Check sheet for the drawn part. Datum: minimum x, y, z corner. Units: mm. A direction names the side the tool comes from. Give positions to 0.01 mm unless a question says otherwise; leave off trailing zeros. Write each loop counter-clockwise with the first axis right and the second up, starting at its lowest first coordinate (ties: lowest second). Pieces come first, ordered by that corner, then holes.
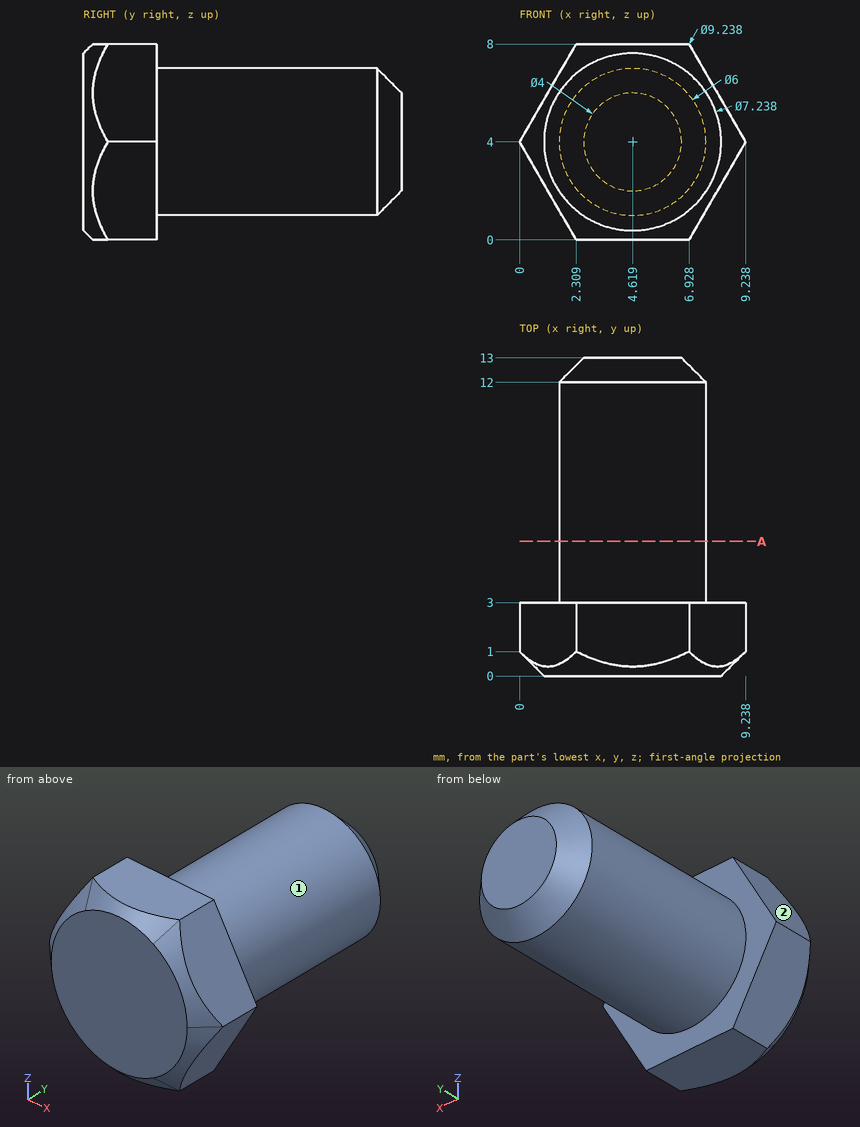
1) Access from +Z, -Z, +X, -X, +Y, -Y to the whole of each face (thin tool, end or side, straight path). Record for the marked faces 1 and 2.
2) Sectioned sample at A-A on y = 5.5. Record the boundary of the cut face in (x, z), then the cut area to 3 significant figures.
3) Scan lines: L1, parallel to Y at x = 4, z = 0.5; L2, parallel to X at y = 12.5, z = 2.5; L3, parallel to Y at x = 6.75, z = 4.5. Record each from-to range of solid material in increasing order.
4) Gauge pin test, flat ends, axial feed: pin 1 (3 mm diameter, centred on x = 2, z = 3, fed in from +Y); pin 2 (2 mm diameter, centred on y = 9.5, z = 3, fed in from -X); pin 3 (2 mm diameter, centred on x = 3.5, y = 7.5, fed in from -Z); pin 4 (2 mm diameter, centred on x = 2, y = 5.5, fed in from -Z) (1 decimal). Record the tip position at first contact, or that the pin passes through.
Answers below:
1. face 1: +Y
1. face 2: +Z, -X, +Y, -Y
2. outline: circle Ø6 at (4.62, 4)
2. area: 28.3 mm2
3. L1: y = 0 to 3
3. L2: x = 2.62 to 6.62
3. L3: y = 0 to 12.81
4. pin 1: stops at y = 13
4. pin 2: stops at x = 1.62
4. pin 3: stops at z = 1
4. pin 4: stops at z = 1.5
